The listing builds one solid part. Answer for the finished solid, in the listing's coordinates (mm). A direction names the side the tool comes from. Give positions to 0.01 mm unless a question says otherwise; leave off trailing zeros. Write each loop counter-clockwise with the first axis right and the second up, starting at its lowest first coordinate (ties: lowest second). Pieces come first, ordered by that corner, then holes.
```python
from build123d import *

# Parameters (mm, degrees)
SKETCH_W     = 73
SKETCH_H     = 10
PAD_DEPTH    = 2
PAD001_DEPTH = 14
SKETCH002_R  = 2
POCKET_DEPTH = 76.201


with BuildPart() as part:
    # Sketch → Pad (new body)
    with BuildSketch(Plane.XY):
        with Locations((0, 5)):
            Rectangle(SKETCH_W, SKETCH_H)
    extrude(amount=PAD_DEPTH)

    # Sketch001 → Pad001 (new body)
    with BuildSketch(Plane(origin=(0, 0, 0), x_dir=(1, 0, 0), z_dir=(0, 0, -1))):
        Polygon((13.5, 1.6), (13.5, 0), (36.5, 0), (36.5, -10), (0, -10), (0, -11.6), (38.1, -11.6), (38.1, 1.6), align=None)
    pad001 = extrude(amount=-PAD001_DEPTH)

    # Mirrored: Pad001 across Sketch001 V_Axis
    add(pad001.mirror(Plane(origin=(0, 0, 0), x_dir=(0, 0, -1), z_dir=(1, 0, 0))))

    # Sketch002 → Pocket (cut, through all)
    with BuildSketch(Plane.YZ.offset(38.1)):
        with Locations((5, 8)):
            Circle(SKETCH002_R)
    extrude(amount=-POCKET_DEPTH, mode=Mode.SUBTRACT)


solid = part.part
```
Item 1: A cutting plane is placed at C-C, the plane x = 19.5. Give the vertices of the cut face in (y, z).
Conclusion:
outline: (-1.6, 0) - (11.6, 0) - (11.6, 14) - (10, 14) - (10, 2) - (0, 2) - (0, 14) - (-1.6, 14) - close
Item 2: Determine the mould class of faces 4 (the face through (-25, 0, 8)), 5 (the face through (0, 11, 14)), 6 (the face through (38.1, 5, 5)), 7 (the face through (-36.5, 7.2, 7.9)) for opening direction X: pulls with the +X half, pulls with the -X half, needs draft (parallel to the pull), parting line crosses it, or undercut.
Conclusion:
face 4: undercut
face 5: needs draft
face 6: pulls with the +X half
face 7: undercut
Item 3: Consider probe 1 along Y at (x, z) = (24, 3); probe 2 along Z at (x, y) = (-37.35, 5); probe 3 along X at (y, z) = (7.5, 9). Determine where each line is inside the solid, lowest interval first.
Conclusion:
probe 1: y = -1.6 to 0, 10 to 11.6
probe 2: z = 0 to 6, 10 to 14
probe 3: x = -38.1 to -36.5, 36.5 to 38.1
Item 4: This flat-tipped pin is pushed along its axis until it touches: P1, Ø1.6, axis at x = -1.5, z = 1, coming from the -Y side. Where does it stop, or does it pass through?
Conclusion:
P1: stops at y = 0
Item 5: A cutting plane is placed at D-D, the plane z = 3. Give the vertices of the cut face in (x, y), plus the area to 3 significant figures.
Conclusion:
outline: (-38.1, -1.6) - (-13.5, -1.6) - (-13.5, 0) - (-36.5, 0) - (-36.5, 10) - (36.5, 10) - (36.5, 0) - (13.5, 0) - (13.5, -1.6) - (38.1, -1.6) - (38.1, 11.6) - (-38.1, 11.6) - close
area: 233 mm2
Item 6: A cutting plane is placed at A-A, the plane y = 5. Give the vertices of the cut face in (x, z), plus the area to 3 significant figures.
Conclusion:
outline: (-38.1, 0) - (38.1, 0) - (38.1, 6) - (36.5, 6) - (36.5, 2) - (-36.5, 2) - (-36.5, 6) - (-38.1, 6) - close; (-38.1, 10) - (-36.5, 10) - (-36.5, 14) - (-38.1, 14) - close; (36.5, 10) - (38.1, 10) - (38.1, 14) - (36.5, 14) - close
area: 178 mm2
Item 7: Which of the six approach directions +Z, -Z, +X, -X, +Y, -Y give full straight-line access (tool end or side, diameter ignored) to faces 1 (the face through (37.311, 3.526, 9.352)), 2 (the face through (-1, 5, 2)), 3 (the face through (0, 0, 1))?
Conclusion:
face 1: +X, -X
face 2: +Z
face 3: +Z, -Z, -Y
Item 8: A cutting plane is placed at B-B, the plane z = 8. Give the vertices of the cut face in (x, y).
Conclusion:
outline: (-38.1, -1.6) - (-13.5, -1.6) - (-13.5, 0) - (-36.5, 0) - (-36.5, 3) - (-38.1, 3) - close; (-38.1, 7) - (-36.5, 7) - (-36.5, 10) - (36.5, 10) - (36.5, 7) - (38.1, 7) - (38.1, 11.6) - (-38.1, 11.6) - close; (13.5, -1.6) - (38.1, -1.6) - (38.1, 3) - (36.5, 3) - (36.5, 0) - (13.5, 0) - close
